Could you check a few things on this drawing? It's one solid part, dimensions in mm from its lowest x, y, z. Give positions to 0.01 mm unless a question says otherwise; leave off trailing zeros. Loops run counter-clockwise (first coordinate to the right, second up) from the corner with the lowest first, then second, coordinate; pieces in that order, holes last. Notation, with made-up numbers: M 38.25,-12 L 44.25,-12 A24 ccw 44.25,17 Z; hole C 88.5,49 d6. An arc over 180 degrees is marked long. Answer as a JSON object with one key per item and string values.
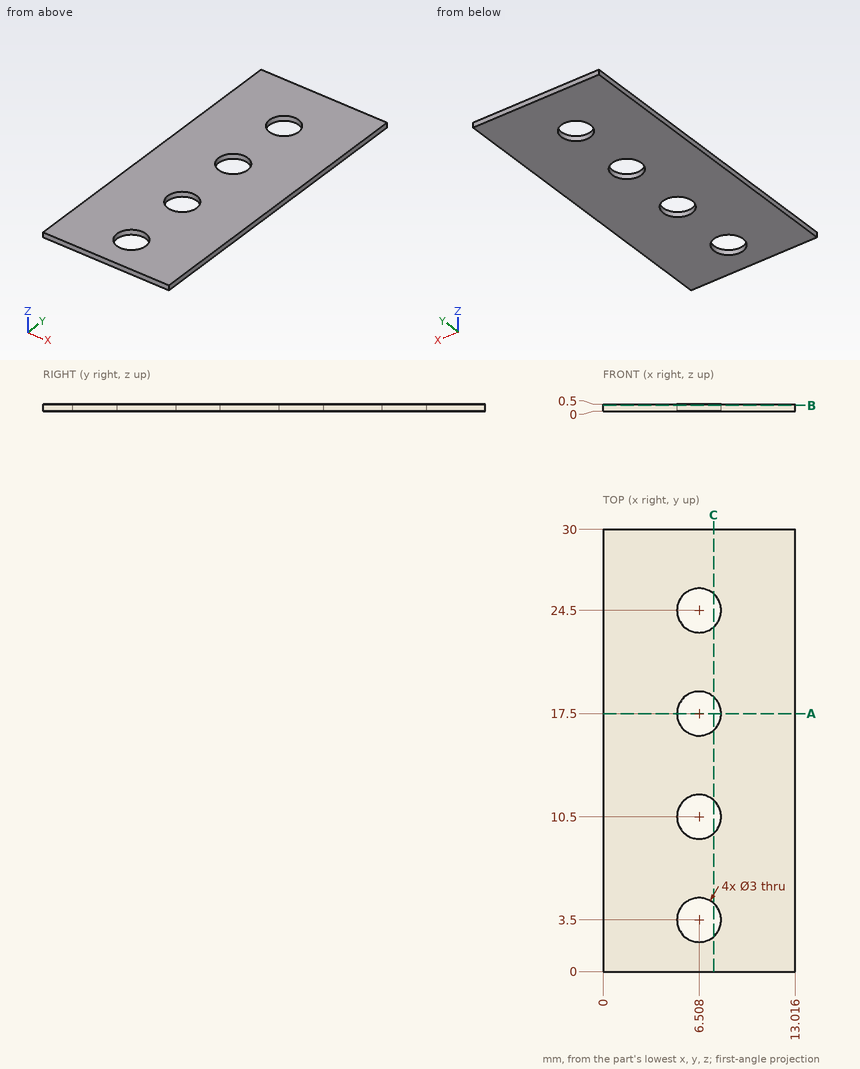
1) Suppose I cut it at C-C, the plane x = 7.5. Write out the boundary of the cut face in (y, z), and give its area (3 significant figures).
Answer list:
{"outline": "M 0,0 L 2.37,0 L 2.37,0.5 L 0,0.5 Z; M 4.63,0 L 9.37,0 L 9.37,0.5 L 4.63,0.5 Z; M 11.63,0 L 16.37,0 L 16.37,0.5 L 11.63,0.5 Z; M 18.63,0 L 23.37,0 L 23.37,0.5 L 18.63,0.5 Z; M 25.63,0 L 30,0 L 30,0.5 L 25.63,0.5 Z", "area": "10.5 mm^2"}
2) Please list where these lines run through material, in increasing order: line 1 along Y through (x, z) = (5.25, 0.3); line 2 along Y through (x, z) = (6.25, 0.3); line 3 along X through (y, z) = (16.75, 0.3). Write a range as from..to.
Answer list:
{"line 1": "0..2.68, 4.32..9.68, 11.32..16.68, 18.32..23.68, 25.32..30", "line 2": "0..2.02, 4.98..9.02, 11.98..16.02, 18.98..23.02, 25.98..30", "line 3": "0..5.21, 7.81..13.02"}
3) Suppose I cut it at B-B, the plane z = 0.4. Write out the boundary of the cut face in (x, y).
Answer list:
{"outline": "M 0,0 L 13.02,0 L 13.02,30 L 0,30 Z; hole C 6.51,3.5 d3; hole C 6.51,10.5 d3; hole C 6.51,17.5 d3; hole C 6.51,24.5 d3"}
4) Will this pin go through, and if not, where does the flat tip stop? pin 1 Ø4 at (x, y) = (5, 20) entering from -Z.
Answer list:
{"pin 1": "z = 0"}
5) Suppose I cut it at A-A, the plane y = 17.5. Write out the boundary of the cut face in (x, z), and give its area (3 significant figures).
Answer list:
{"outline": "M 0,0 L 5.01,0 L 5.01,0.5 L 0,0.5 Z; M 8.01,0 L 13.02,0 L 13.02,0.5 L 8.01,0.5 Z", "area": "5.01 mm^2"}
